The model under review builds one solid part; all positions refer to its coordinate system, in mm. Face numbers are marked on the shaded views. Give positions to 0.01 mm unless a question says otherwise; leave off trailing zeros. Order: outer loops, then holes, each group sorted by start corner. A loop starts at its lowest first (then second) coordinate and runs counter-clockwise, first axis right, second up. Notation, with made-up numbers: (21.5, 61.5) -> (35.5, 61.5) arc R18 ccw to (35.5, 79.5) -> close; hole circle Ø10 at (6.5, 45.25). An arc over 180 degrees is marked (long way). Answer as a JSON object with one key per item and string values. Group by question number.
from build123d import *

# Parameters (mm, degrees)
SKETCH_1_R               = 10
SKETCH_1_R_2             = 6
EXTRUDE_1_DEPTH          = 120
CUT_EXTRUDE_1_DEPTH      = 121.830459736
CUT_EXTRUDE_1_DEPTH_BACK = 121.830459736
SKETCH_2_R               = 1.65


with BuildPart() as part:
    # Эскиз1 → Бобышка-Вытянуть1 (new body)
    with BuildSketch(Plane.XY):
        Circle(SKETCH_1_R)
        Circle(SKETCH_1_R_2, mode=Mode.SUBTRACT)
    extrude(amount=EXTRUDE_1_DEPTH)

    # Эскиз2 → Вырез-Вытянуть1 (cut, two sides: drawn at the far end of the back side and taken through both)
    with BuildSketch(Plane(origin=(0, 0, 0), x_dir=(1, 0, 0), z_dir=(0, 1, 0)).offset(-CUT_EXTRUDE_1_DEPTH_BACK)):
        with Locations(Location((0, -10.65, 0), (0, 0, 270))):
            Circle(SKETCH_2_R)
        with Locations(Location((0, -59.65, 0), (0, 0, 270))):
            Circle(SKETCH_2_R)
    extrude(amount=CUT_EXTRUDE_1_DEPTH + CUT_EXTRUDE_1_DEPTH_BACK, mode=Mode.SUBTRACT)


solid = part.part
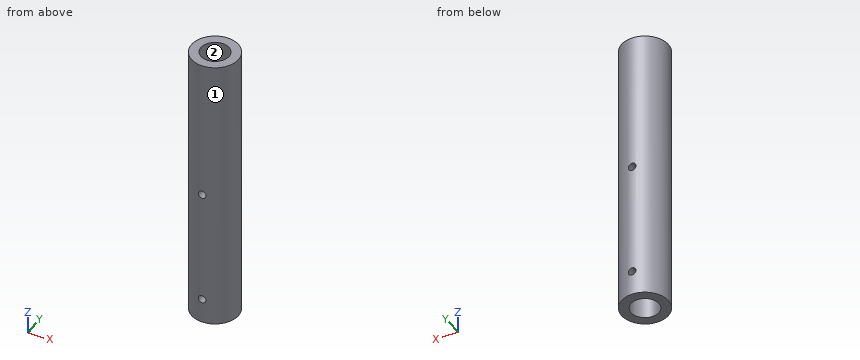
1. Take a section at B-B on x = 0. Give the boundary of the cut face in (y, z), plus the area to 3 significant figures.
2. For pin 1 (1.5 mm diameter, centred on y = 2.5, z = 88.5, fed in from +X); pin 2 (2.5 mm diameter, centred on x = 0, z = 59.65, fed in from -Y); pin 3 (8 mm diameter, centred on y = -7, z = 107.5, fed in from -X); pin 4 (1.5 mm diameter, centred on y = 2.5, z = 37.5, fed in from -X), all flat-tipped, find the tip position at first contact; note any pin that passes through.
3. Draft analysis for pull direction Y (two halves, no side actions). For the marked faces 1 and 2, state which applies: pulls with the +Y half, pulls with the -Y half, needs draft (parallel to the pull), parting line crosses it, or undercut.
4. For probe 1 along Z at (x, y) = (0, -7.25); probe 2 along Y at (x, z) = (-0.5, 95.5); probe 3 along Z at (x, y) = (-1.5, 6), list the stretches that pass through material, from the lowest coordinate up. Write a range as [from, to].
5. Take a section at C-C on z = 59.65. Give the boundary of the cut face in (x, y).
6. Take a section at A-A on y = 0. Give the boundary of the cut face in (x, z), plus the area to 3 significant figures.
7. Take a section at D-D on y = -7.75. Give the boundary of the cut face in (x, z), plus the area to 3 significant figures.
Checks:
{
 "1": {"outline": "(-10, 0) -> (-6, 0) -> (-6, 9) -> (-10, 9) -> close; (-10, 12.3) -> (-6, 12.3) -> (-6, 58) -> (-10, 58) -> close; (-10, 61.3) -> (-6, 61.3) -> (-6, 120) -> (-10, 120) -> close; (6, 0) -> (10, 0) -> (10, 9) -> (6, 9) -> close; (6, 12.3) -> (10, 12.3) -> (10, 58) -> (6, 58) -> close; (6, 61.3) -> (10, 61.3) -> (10, 120) -> (6, 120) -> close", "area": "907 mm2"},
 "2": {"pin 1": "stops at x = 9.85", "pin 2": "passes through", "pin 3": "stops at x = -9.54", "pin 4": "stops at x = -9.85"},
 "3": {"face 1": "parting line crosses it", "face 2": "undercut"},
 "4": {"probe 1": "z = [0, 9], [12.3, 58], [61.3, 120]", "probe 2": "y = [-9.99, -5.98], [5.98, 9.99]", "probe 3": "z = [0, 9.96], [11.34, 58.96], [60.34, 120]"},
 "5": {"outline": "(-1.65, -9.86) -> (-1.65, -5.77) arc R6 cw to (-1.65, 5.77) -> (-1.65, 9.86) arc R10 ccw to start; (1.65, -9.86) arc R10 ccw to (1.65, 9.86) -> (1.65, 5.77) arc R6 cw to (1.65, -5.77) -> close"},
 "6": {"outline": "(-10, 0) -> (-6, 0) -> (-6, 120) -> (-10, 120) -> close; (6, 0) -> (10, 0) -> (10, 120) -> (6, 120) -> close", "area": "960 mm2"},
 "7": {"outline": "(-6.32, 0) -> (6.32, 0) -> (6.32, 120) -> (-6.32, 120) -> close; hole circle Ø3.3 at (0, 10.65); hole circle Ø3.3 at (0, 59.65)", "area": "1,500 mm2"}
}
